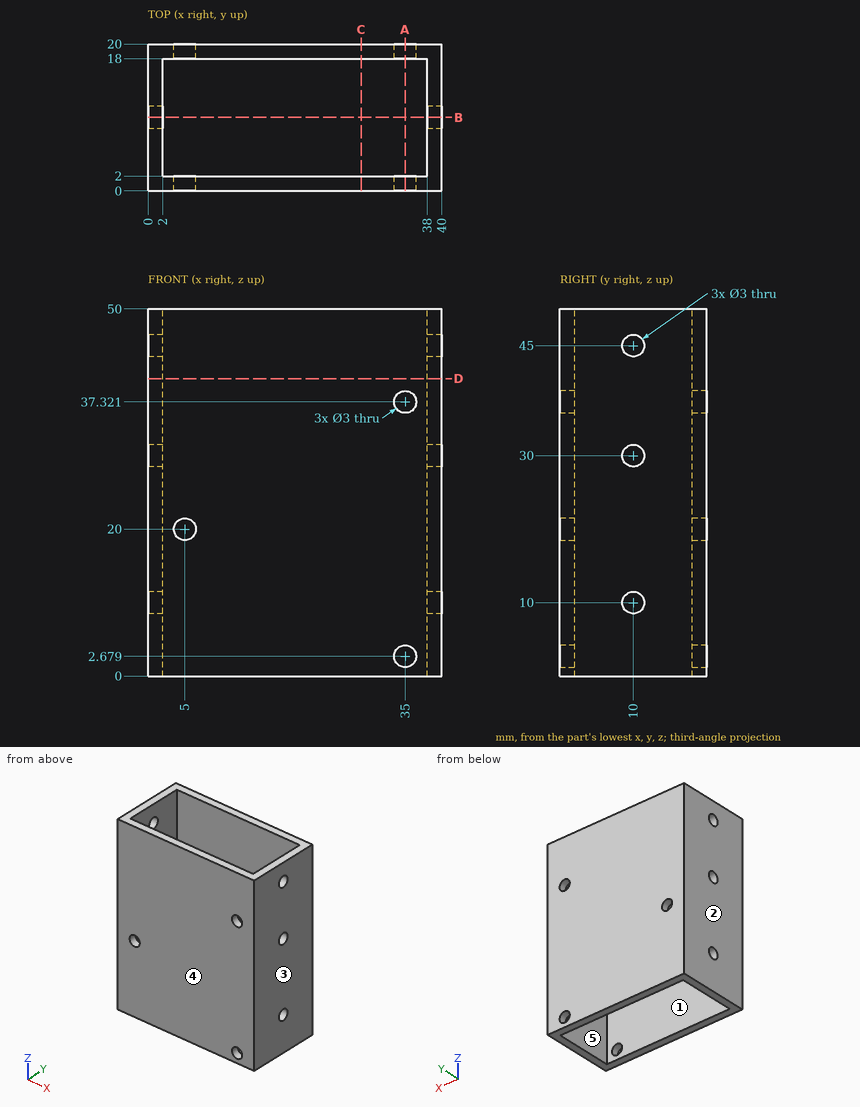
The figure shows three views and two pictorial views of one solid part (mm, origin at its lowest corner). Answer the questions. A direction names the side the tool comes from. Round coordinates to 2 decimals unless told otherwise and drop trailing zeros. Order: outer loops, then holes, each group sorted by start corner. A loop starts at its lowest first (then second) coordinate and runs counter-clockwise, first axis right, second up.
Q1. Find the intervals of material crossed by line 1 along Y through (x, z) = (19.5, 22); line 2 along X through (y, z) = (9.5, 31.5), in increasing order.
Solution:
line 1: y = 0 to 2, 18 to 20
line 2: x = 0 to 2, 38 to 40
Q2. A cutting plane is placed at A-A, the plane x = 35. Determine the outline of the cut face in (y, z).
Solution:
outline: (0, 0) - (2, 0) - (2, 1.18) - (0, 1.18) - close; (0, 4.18) - (2, 4.18) - (2, 35.82) - (0, 35.82) - close; (0, 38.82) - (2, 38.82) - (2, 50) - (0, 50) - close; (18, 0) - (20, 0) - (20, 1.18) - (18, 1.18) - close; (18, 4.18) - (20, 4.18) - (20, 35.82) - (18, 35.82) - close; (18, 38.82) - (20, 38.82) - (20, 50) - (18, 50) - close
Q3. A cutting plane is placed at B-B, the plane y = 10. Count the separate pieces of the cut face and the enclosed holes in it, then the cut area to 3 significant figures.
Solution:
separate pieces: 8
enclosed holes: 0
area: 164 mm2
Q4. The mould has two halves that part along Y. Classify the marked faces 3, 4 and 5: pulls with the +Y half, pulls with the -Y half, needs draft (parallel to the pull), parting line crosses it, or undercut.
Solution:
face 3: needs draft
face 4: pulls with the -Y half
face 5: undercut
Q5. A cutting plane is placed at D-D, the plane z = 40.5. Determine the outline of the cut face in (x, y), then the cut area to 3 significant figures.
Solution:
outline: (0, 0) - (40, 0) - (40, 20) - (0, 20) - close; hole (2, 2) - (38, 2) - (38, 18) - (2, 18) - close
area: 224 mm2
Q6. A tool of negligible diameter and unlimited length cuts with its end or side. For the marked faces 1 and 2, from which of +Z, -Z, +X, -X, +Y, -Y can it reach the whole face along a straight path? Write none if from no direction.
Solution:
face 1: +Z, -Z
face 2: +Z, -Z, -X, +Y, -Y
Q7. A cutting plane is placed at C-C, the plane x = 29. Determine the outline of the cut face in (y, z).
Solution:
outline: (0, 0) - (2, 0) - (2, 50) - (0, 50) - close; (18, 0) - (20, 0) - (20, 50) - (18, 50) - close
